from build123d import *

# Parameters (mm, degrees)
BOSS_EXTRUDE1_DEPTH = 100
FILLET1_R           = 50
SKETCH2_R           = 5
CUT_EXTRUDE1_DEPTH  = 116
SKETCH5_W           = 116
SKETCH5_H           = 120
BOSS_EXTRUDE4_DEPTH = 8
SKETCH6_W           = 100
SKETCH6_H           = 120
BOSS_EXTRUDE6_DEPTH = 8


with BuildPart() as part:
    # Sketch1 → Boss-Extrude1 (new body)
    with BuildSketch(Plane.XY):
        Polygon((8, -171), (8, -8), (8, 0), (0, 0), (0, -8), (0, -146), (0, -154), (0, -292), (0, -350), (8, -350), (8, -292), (8, -179), (108, -179), (108, -292), (108, -350), (116, -350), (116, -292), (116, -154), (116, -146), (116, -8), (116, 0), (108, 0), (108, -8), (108, -171), align=None)
    extrude(amount=BOSS_EXTRUDE1_DEPTH)

    # Fillet1
    fillet1_edges = [part.edges().sort_by_distance(p)[0] for p in [
        (4, 0, 100),
        (4, 0, 0),
        (112, -350, 0),
        (112, -350, 100),
        (4, -350, 100),
        (4, -350, 0),
        (112, 0, 100),
        (112, 0, 0),
    ]]
    fillet(fillet1_edges, radius=FILLET1_R - 0.0001)  # a hair under: the kernel refuses the full size

    # Sketch2 → Cut-Extrude1 (cut)
    with BuildSketch(Plane(origin=(116, 0, 0), x_dir=(0, 0, -1), z_dir=(1, 0, 0))):
        with Locations(Location((-50, -300, 0), (0, 0, 90))):
            Circle(SKETCH2_R)
        with Locations(Location((-50, -50, 0), (0, 0, 90))):
            Circle(SKETCH2_R)
    extrude(amount=-CUT_EXTRUDE1_DEPTH, mode=Mode.SUBTRACT)

    # Sketch5 → Boss-Extrude4 (add)
    with BuildSketch(Plane.XY.offset(100)):
        with Locations((58, -175)):
            Rectangle(SKETCH5_W, SKETCH5_H)
    extrude(amount=-BOSS_EXTRUDE4_DEPTH)

    # Sketch6 → Boss-Extrude6 (add)
    with BuildSketch(Plane(origin=(0, 0, 0), x_dir=(-1, 0, 0), z_dir=(0, 0, -1))):
        with Locations((-58, -175)):
            Rectangle(SKETCH6_W, SKETCH6_H)
    extrude(amount=-BOSS_EXTRUDE6_DEPTH)


solid = part.part
Design review of the part built by this model. Coordinates are the model's own, in mm. A direction names the side the tool comes from. Round coordinates to 2 decimals unless told otherwise and drop trailing zeros. Write each loop counter-clockwise with the first axis right and the second up, starting at its lowest first coordinate (ties: lowest second). Pieces come first, ordered by that corner, then holes. Notation, with made-up numbers: M 56.5,-31.5 L 82.5,-31.5 A14 ccw 82.5,-23.5 Z; hole C 49,5.25 d10. An arc over 180 degrees is marked long. One line per item, written item: value. Start each with the question number.
1. Take a section at A-A on y = -111.5. State the section outline as (x, z) points.
2. Take a section at B-B on x = 99.5. State the section outline as (y, z) points, then the cut area to 3 significant figures.
3. To check wall thickness, follow probe 1 along X at (y, z) = (-158, 85.5); probe 2 along Z at (x, y) = (97, -183.5); probe 3 along Y at (x, z) = (47, 67). State the ranges of each line that lie inside material, in increasing order. Write a range as from..to.
4. Take a section at C-C on y = -212. State the section outline as (x, z) points.
5. Draft analysis for pull direction Z (two halves, no side actions). For faces 4 (the face through (112.06, -295.23, 51.5)), 5 (the face through (112.056, -335.742, 84.964)), 6 (the face through (57, -115, 96)), state which applies: pulls with the +Z half, pulls with the -Z half, needs draft (parallel to the pull), parting line crosses it, or undercut.
6. Clearance check with flat-ended pins moving along their axes: P1, Ø6.5, axis at x = 48.5, z = 96.5, coming from the -Y side; P2, Ø5, axis at x = 98.5, z = 14.5, coming from the -Y side; P3, Ø4, axis at x = 44.5, z = 4, coming from the +Y side; P4, Ø9, axis at y = -300, z = 50, coming from the -X side. State where each tip first meets the part, or that it passes through.
7. For faces 1 (the face through (108, -84, 49)), 2 (the face through (112.056, -335.742, 15.036)), 3 (the face through (57, -207, 92)), list the 3-axis set-ups (+Z, -Z, +X, -X, +Y, -Y) from which the entire face can be reached by the end or side of a thin tool; tool diameter is ignored.
8. Take a section at D-D on z = 28.5. State the section outline as (x, y) points.
Computed:
1. outline: M 0,0 L 8,0 L 8,100 L 0,100 Z; M 108,0 L 116,0 L 116,100 L 108,100 Z
2. outline: M -235,0 L -115,0 L -115,8 L -171,8 L -171,92 L -115,92 L -115,100 L -235,100 L -235,92 L -179,92 L -179,8 L -235,8 Z
2. area: 2,590 mm²
3. probe 1: x = 0..8, 108..116
3. probe 2: z = 0..8, 92..100
3. probe 3: y = -179..-171
4. outline: M 0,0 L 116,0 L 116,100 L 0,100 Z; hole M 8,8 L 108,8 L 108,92 L 8,92 Z
5. face 4: undercut
5. face 5: pulls with the +Z half
5. face 6: needs draft
6. P1: stops at y = -235
6. P2: stops at y = -179
6. P3: stops at y = -115
6. P4: passes through
7. face 1: +Y
7. face 2: -Z, +X, -X, -Y
7. face 3: -Y
8. outline: M 0,-345.14 L 8,-345.14 L 8,-179 L 108,-179 L 108,-345.14 L 116,-345.14 L 116,-4.86 L 108,-4.86 L 108,-171 L 8,-171 L 8,-4.86 L 0,-4.86 Z
